```python
from build123d import *

# Parameters (mm, degrees)
SKETCH1_W           = 1010
SKETCH1_H           = 775
BOSS_EXTRUDE1_DEPTH = 4
FILLET1_R           = 20
SKETCH2_W           = 500
SKETCH2_H           = 100
SKETCH2_W_2         = 80
CUT_EXTRUDE1_DEPTH  = 10
FILLET2_R           = 20


with BuildPart() as part:
    # Sketch1 → Boss-Extrude1 (new body)
    with BuildSketch(Plane.XY):
        Rectangle(SKETCH1_W, SKETCH1_H)
    extrude(amount=BOSS_EXTRUDE1_DEPTH)

    # Fillet1
    fillet1_edges = [part.edges().sort_by_distance(p)[0] for p in [
        (505, -387.5, 2),
        (-505, -387.5, 2),
        (-505, 387.5, 2),
        (505, 387.5, 2),
    ]]
    fillet(fillet1_edges, radius=FILLET1_R)

    # Sketch2 → Cut-Extrude1 (cut)
    with BuildSketch(Plane.XY.offset(4)):
        Polygon((60, 230), (250, 230), (330, 230), (330, 387.5), (60, 387.5), align=None)
        with Locations((0, 180)):
            Rectangle(SKETCH2_W, SKETCH2_H)
        with Locations((290, 180)):
            Rectangle(SKETCH2_W_2, SKETCH2_H)
    extrude(amount=-CUT_EXTRUDE1_DEPTH, mode=Mode.SUBTRACT)

    # Fillet2
    fillet2_edges = [part.edges().sort_by_distance(p)[0] for p in [
        (60, 387.5, 2),
        (330, 387.5, 2),
        (330, 130, 2),
        (-250, 130, 2),
        (-250, 230, 2),
        (60, 230, 2),
    ]]
    fillet(fillet2_edges, radius=FILLET2_R)


solid = part.part
```
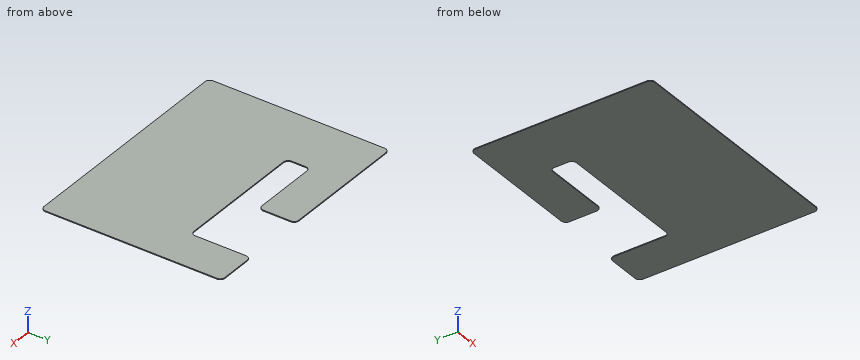
Verification items for the finished model (mm, model axes). Give positions to 0.01 mm unless a question says otherwise; leave off trailing zeros. Order: outer loops, then holes, each group sorted by start corner. A loop starts at its lowest first (then second) coordinate and runs counter-clockwise, first axis right, second up. Notation, with made-up numbers: (-8, 28.5) -> (13, 28.5) arc R18 cw to (13, 43.5) -> close; hole circle Ø3 at (31.25, 71). An arc over 180 degrees is marked (long way). Use a Markdown table: item, result.
1) Material ranges on probe 1 along X at (y, z) = (187.5, 1.3); probe 2 along X at (y, z) = (275, 1.25); probe 3 along Y at (x, z) = (245.5, 0.65), recorded low to high.
Results:
| item | result |
|---|---|
| probe 1 | -505 to -250, 330 to 505 |
| probe 2 | -505 to 60, 330 to 505 |
| probe 3 | -387.5 to 130 |
2) Section check B-B, the plane x = -142. Record the boundary of the cut face in (y, z), then the cut area to 3 significant figures.
Results:
| item | result |
|---|---|
| outline | (-387.5, 0) -> (130, 0) -> (130, 4) -> (-387.5, 4) -> close; (230, 0) -> (387.5, 0) -> (387.5, 4) -> (230, 4) -> close |
| area | 2,700 mm² |
3) Section check A-A, the plane y = 320. Record the boundary of the cut face in (x, z), then the cut area to 3 significant figures.
Results:
| item | result |
|---|---|
| outline | (-505, 0) -> (60, 0) -> (60, 4) -> (-505, 4) -> close; (330, 0) -> (505, 0) -> (505, 4) -> (330, 4) -> close |
| area | 2,960 mm² |
4) Depth check by flat-ended pin: pin 1 Ø1.2 at (x, z) = (133.5, 2) entering from +Y. Enter the tip coordinate at first touch or a pass-through.
Results:
| item | result |
|---|---|
| pin 1 | y = 130 |
5) Section check C-C, the plane z = 1.4. Record the boundary of the cut face in (x, y), then the cut area to 3 significant figures.
Results:
| item | result |
|---|---|
| outline | (-505, -367.5) arc R20 ccw to (-485, -387.5) -> (485, -387.5) arc R20 ccw to (505, -367.5) -> (505, 367.5) arc R20 ccw to (485, 387.5) -> (350, 387.5) arc R20 ccw to (330, 367.5) -> (330, 150) arc R20 cw to (310, 130) -> (-230, 130) arc R20 cw to (-250, 150) -> (-250, 210) arc R20 cw to (-230, 230) -> (40, 230) arc R20 ccw to (60, 250) -> (60, 367.5) arc R20 ccw to (40, 387.5) -> (-485, 387.5) arc R20 ccw to (-505, 367.5) -> close |
| area | 682,000 mm² |
6) Section check D-D, the plane x = 179. Record the boundary of the cut face in (y, z), then the cut area to 3 significant figures.
Results:
| item | result |
|---|---|
| outline | (-387.5, 0) -> (130, 0) -> (130, 4) -> (-387.5, 4) -> close |
| area | 2,070 mm² |
